from build123d import *

# Parameters (mm, degrees)
ESBO_O2_R                  = 4.9
CORTE_EXTRUS_O1_DEPTH      = 10
CHANFRO1_SIZE              = 0.5
CORTE_EXTRUS_O2_DEPTH      = 62.23724357
CORTE_EXTRUS_O2_DEPTH_BACK = 62.23724357
ESBO_O3_W                  = 5
ESBO_O3_H                  = 20
FILETE1_R                  = 5


with BuildPart() as part:
    # Esboço1 → Revolução1 (revolve)
    with BuildSketch(Plane.XY):
        Polygon((0, 0), (-25, 0), (-25, 50), (-12.5, 50), (-12.5, 10), (0, 10), align=None)
    revolve(axis=Axis((0, 10, 0), (0, -1, 0)))

    # Esboço2 → Corte-extrusão1 (cut)
    with BuildSketch(Plane(origin=(0, 10, 0), x_dir=(1, 0, 0), z_dir=(0, 1, 0))):
        with Locations(Location((0, 7, 0), (0, 0, 180))):
            Circle(ESBO_O2_R)
        with Locations(Location((0, -7, 0), (0, 0, 180))):
            Circle(ESBO_O2_R)
    extrude(amount=-CORTE_EXTRUS_O1_DEPTH, mode=Mode.SUBTRACT)

    # Chanfro1
    chanfro1_edges = [part.edges().sort_by_distance(p)[0] for p in [
        (4.9, 0, -7),
        (4.9, 0, 7),
    ]]
    chamfer(chanfro1_edges, length=CHANFRO1_SIZE)

    # Esboço3 → Corte-extrusão2 (cut, two sides: drawn at the far end of the back side and taken through both)
    with BuildSketch(Plane.XY.offset(-CORTE_EXTRUS_O2_DEPTH_BACK)):
        with Locations((-22.5, 10)):
            Rectangle(ESBO_O3_W, ESBO_O3_H)
        with Locations((22.5, 10)):
            Rectangle(ESBO_O3_W, ESBO_O3_H)
    extrude(amount=CORTE_EXTRUS_O2_DEPTH + CORTE_EXTRUS_O2_DEPTH_BACK, mode=Mode.SUBTRACT)

    # Filete1
    filete1_edges = [part.edges().sort_by_distance(p)[0] for p in [
        (20, 20, 0),
        (-20, 20, 0),
    ]]
    fillet(filete1_edges, radius=FILETE1_R - 0.0001)  # a hair under: the kernel refuses the full size


solid = part.part
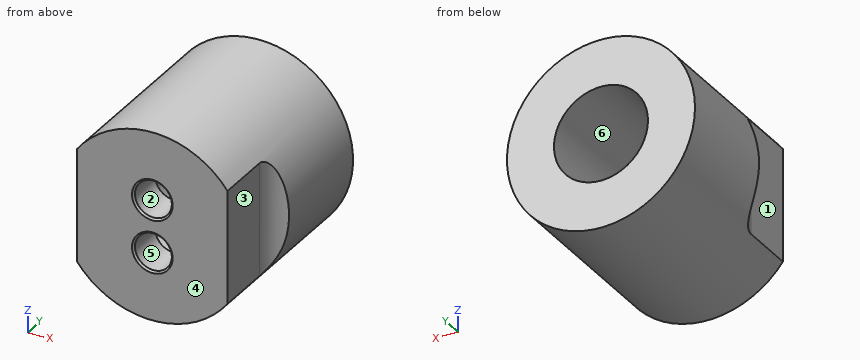
For this review, take the finished solid that the model builds, in its own axes (mm). Face numbers are marked on the shaded views. A direction names the side the tool comes from. Round coordinates to 2 decimals unless told otherwise and drop trailing zeros. Order: outer loops, then holes, each group sorted by start corner. A loop starts at its lowest first (then second) coordinate and runs counter-clockwise, first axis right, second up. Notation, with made-up numbers: M -2,16 L 23,16 A12 ccw 23,39 Z; hole C 84.5,-8 d7. An arc over 180 degrees is marked long. Use a Markdown table: item, result. Add a question column.
Item 1: To check wall thickness, follow line 1 along Z through (x, y) = (0, 3); line 2 along Z through (x, y) = (0, 32); line 3 along Z through (x, y) = (7, 23.5). State the ranges of each line that lie inside material, in increasing order.
Item 2: Insertion check: pin 1 (7.5 mm diameter, centred on y = 5, z = 3, fed in from +X); pin 2 (3 mm diameter, centred on y = 16.5, z = -18, fed in from +X); pin 3 (1.5 mm diameter, centred on x = -7.5, y = 18, fed in from -Z); pin 4 (6 mm diameter, centred on x = 0, z = 7, fed in from +Y). Each pin has a flat end and moves straight along its axis. Give the tip position at first contact, or say it passes through.
Item 3: Add section B-B, the plane y = 14. Give the boundary of the cut face in (x, z), then the cut area to 3 significant figures.
Item 4: Mouldability with a two-part tool opening along X and no side actions: class the marked faces 3, 4, 5 and 6 as released by +X, released by -X, zero draft, split by the parting line, or undercut.
Item 5: Add section A-A, the plane x = 0. Give the boundary of the cut face in (y, z), then the cut area to 3 significant figures.
Item 6: Add section C-C, the plane z = -7. Give the boundary of the cut face in (x, y), then the cut area to 3 significant figures.
Item 7: Tool access review of the marked faces 1 and 2: name each direction out of +Z, -Z, +X, -X, +Y, -Y from which nothing blocks a thin tool from reaching the whole face with its end or side.
Item 8: Add section D-D, the plane x = 6.5. Give the boundary of the cut face in (y, z).
Geometry results:
| question | item | result |
|---|---|---|
| 1 | line 1 | z = -25 to -11.9, -2.1 to 2.1, 11.9 to 25 |
| 1 | line 2 | z = -25 to -12.5, 12.5 to 25 |
| 1 | line 3 | z = -24 to -10.36, 10.36 to 24 |
| 2 | pin 1 | stops at x = 20 |
| 2 | pin 2 | stops at x = 18.78 |
| 2 | pin 3 | stops at z = -24.07 |
| 2 | pin 4 | passes through |
| 3 | outline | M -20,-15 A25 ccw 20,-15 L 20,15 A25 ccw -20,15 Z; hole C 0,0 d25 |
| 3 | area | 1,270 mm² |
| 4 | face 3 | released by +X |
| 4 | face 4 | zero draft |
| 4 | face 5 | undercut |
| 4 | face 6 | undercut |
| 5 | outline | M 0,-25 L 50,-25 L 50,-12.5 L 10,-12.5 L 10,-11.9 L 0.5,-11.9 L 0,-12.4 Z; M 0,-1.6 L 0.5,-2.1 L 10,-2.1 L 10,2.1 L 0.5,2.1 L 0,1.6 Z; M 0,12.4 L 0.5,11.9 L 10,11.9 L 10,12.5 L 50,12.5 L 50,25 L 0,25 Z |
| 5 | area | 1,300 mm² |
| 6 | outline | M -24,19.9 A5 cw -20,15 L -20,0 L -5.4,0 L -4.9,0.5 L -4.9,10 L -10.36,10 L -10.36,50 L -24,50 Z; M 4.9,0.5 L 5.4,0 L 20,0 L 20,15 A5 cw 24,19.9 L 24,50 L 10.36,50 L 10.36,10 L 4.9,10 Z |
| 6 | area | 1,320 mm² |
| 7 | face 1 | +Z, -Z, -X, -Y |
| 7 | face 2 | +Y, -Y |
| 8 | outline | M 0,-24.14 L 50,-24.14 L 50,-10.68 L 10,-10.68 L 10,10.68 L 50,10.68 L 50,24.14 L 0,24.14 Z |
